Design review of the part built by this model. Coordinates are the model's own, in mm. A direction names the side the tool comes from. Coordinates: 2 decimals unless noted, no trailing zeros. Order: outer loops, then holes, each group sorted by start corner. A loop starts at its lowest first (then second) coordinate and runs counter-clockwise, first axis right, second up. Notation, with made-up numbers: (66, 45.25) - (99, 45.25) arc R14 ccw to (99, 53.25) - close; hole circle Ø6 at (68.25, 59.25). An arc over 180 degrees is marked (long way). Write item = value, one per line. Start each with the question number.
```python
from build123d import *

# Parameters (mm, degrees)
BASE_FLANGE1_DEPTH = 40
FILLET1_R          = 10
SKETCH6_R          = 4.25
CUT_EXTRUDE1_DEPTH = 88.863530546


# Sheet-metal steps are written as plain solids
with BuildPart() as part:
    # Sketch1 → Base-Flange1 (new body)
    with BuildSketch(Plane.XY):
        with BuildLine():
            Line((0, 0), (0, 38.2634))
            ThreePointArc((0, 38.2634), (0.215745145, 38.784254855), (0.7366, 39))
            Line((0.7366, 39), (59.2634, 39))
            ThreePointArc((59.2634, 39), (59.784254855, 38.784254855), (60, 38.2634))
            Line((60, 38.2634), (60, 0))
            Line((60, 0), (63, 0))
            Line((63, 0), (63, 38.2634))
            ThreePointArc((63, 38.2634), (61.905575199, 40.905575199), (59.2634, 42))
            Line((59.2634, 42), (0.7366, 42))
            ThreePointArc((0.7366, 42), (-1.905575199, 40.905575199), (-3, 38.2634))
            Line((-3, 38.2634), (-3, 0))
            Line((-3, 0), (0, 0))
        make_face()
    extrude(amount=-BASE_FLANGE1_DEPTH)

    # Fillet1
    fillet1_edges = [part.edges().sort_by_distance(p)[0] for p in [
        (-1.5, 0, 0),
        (61.5, 0, 0),
        (-1.5, 0, -40),
        (61.5, 0, -40),
    ]]
    fillet(fillet1_edges, radius=FILLET1_R)

    # Sketch6 → Cut-Extrude1 (cut, through all)
    with BuildSketch(Plane.ZY.offset(3)):
        with Locations((-20, 17)):
            Circle(SKETCH6_R)
    extrude(amount=-CUT_EXTRUDE1_DEPTH, mode=Mode.SUBTRACT)


solid = part.part
```
Item 1: For P1, Ø5, axis at x = 30, z = -35, coming from the -Y side, flat-tipped, find the tip position at first contact; note if it passes through.
Item 2: Add section B-B on z = -20. Give the boundary of the cut face in (x, y), plus the area to 3 significant figures.
Item 3: Add section D-D on x = 28. Give the boundary of the cut face in (y, z), plus the area to 3 significant figures.
Item 4: Add section C-C on y = 17. Give the boundary of the cut face in (x, z), plus the area to 3 significant figures.
Item 5: For line 1 (X direction, y = 30, z = -24.5); line 2 (Y direction, x = 25.5, z = -20); line 3 (Y direction, x = 61.85, z = -20), list the stretches that pass through material, from the lowest coordinate up.
Item 6: Add section A-A on y = 4. Give the boundary of the cut face in (x, z).
Item 7: For faces 1 (the flat face through (30, 40, 0)), 2 (the flat face through (30, 39, -20)), list the 3-axis set-ups (+Z, -Z, +X, -X, +Y, -Y) from which the entire face can be reached by the end or side of a thin tool; tool diameter is ignored.
Item 8: Mouldability with a two-part tool opening along Y and no side actions: class faces 3 (the cylindrical face through (-1.88, 40.93, -19.72)), 4 (the cylindrical face through (-1.52, 12.85, -20.92)), 5 (the flat face through (63, 23, -20)) as +Y half, -Y half, draft (parallel to the pull), parting line (faces both ways), or undercut.
Worked out:
q1.P1 = 39
q2.outline = (-3, 0) - (0, 0) - (0, 12.75) - (-3, 12.75) - close; (-3, 21.25) - (0, 21.25) - (0, 38.26) arc R0.74 cw to (0.74, 39) - (59.26, 39) arc R0.74 cw to (60, 38.26) - (60, 21.25) - (63, 21.25) - (63, 38.26) arc R3.74 ccw to (59.26, 42) - (0.74, 42) arc R3.74 ccw to (-3, 38.26) - close; (60, 0) - (63, 0) - (63, 12.75) - (60, 12.75) - close
q2.area = 375 mm2
q3.outline = (39, -40) - (42, -40) - (42, 0) - (39, 0) - close
q3.area = 120 mm2
q4.outline = (-3, -40) - (0, -40) - (0, -24.25) - (-3, -24.25) - close; (-3, -15.75) - (0, -15.75) - (0, 0) - (-3, 0) - close; (60, -40) - (63, -40) - (63, -24.25) - (60, -24.25) - close; (60, -15.75) - (63, -15.75) - (63, 0) - (60, 0) - close
q4.area = 189 mm2
q5.line_1 = -3 to 0, 60 to 63
q5.line_2 = 39 to 42
q5.line_3 = 0 to 12.75, 21.25 to 40.96
q6.outline = (-3, -38) - (0, -38) - (0, -2) - (-3, -2) - close; (60, -38) - (63, -38) - (63, -2) - (60, -2) - close
q7.face_1 = +Z, +X, -X, +Y, -Y
q7.face_2 = +Z, -Z, -Y
q8.face_3 = +Y half
q8.face_4 = undercut
q8.face_5 = draft
